Autodesk Inventor part; units mm, degrees
ref_plane "YZ Plane" through (0, 0, 0) normal (1, 0, 0) x (0, 1, 0)
ref_plane "XZ Plane" through (0, 0, 0) normal (0, 1, 0) x (-1, 0, 0)
ref_plane "XY Plane" through (0, 0, 0) normal (0, 0, 1) x (1, 0, 0)
sketch "スケッチ1" plane through (0, 0, 0) normal (0, 0, 1) x (1, 0, 0)
  line L0 (-20, -5) -> (20, -5)
  line L1 (20, -5) -> (20, 5)
  line L2 (20, 5) -> (-20, 5)
  line L3 (-20, 5) -> (-20, -5)
  line L4 (-20, -5) -> (20, 5) construction
  line L5 (20, -5) -> (-20, 5) construction
  point P0 (0, 0)
  dimension "d0" = 40
  dimension "d1" = 10
extrude "押し出し1" add sketch "スケッチ1" along normal mid plane 3
sketch "スケッチ2" plane through (-20, -5, 1.5) normal (-1, 0, 0) x (0, 0, 1)
  line L0 (0, 0) -> (0, 10)
  line L1 (-3, 3) -> (0, 3)
  line L2 (0, 3) -> (0, 7)
  line L3 (0, 7) -> (-3, 7)
  line L4 (-3, 7) -> (-3, 3)
  line L5 (-3, 3) -> (0, 7) construction
  line L6 (0, 3) -> (-3, 7) construction
  point P0 (-1.5, 5)
  dimension "d4" = 4
extrude "押し出し2" add sketch "スケッチ2" along normal blind 5
sketch "スケッチ3" plane through (20, -5, 1.5) normal (1, 0, 0) x (0, 0, -1)
  line L0 (3, 7) -> (0, 7)
  line L1 (0, 3) -> (3, 3)
  line L2 (3, 10) -> (0, 10)
  line L3 (0, 0) -> (0, 10)
  line L4 (0, 0) -> (3, 0)
  line L5 (3, 10) -> (3, 0)
  point P0 (1.5, 5)
extrude "押し出し3" add sketch "スケッチ3" along normal blind 5 contours L5 L1 L3 L0
fillet "フィレット1" radius 1 8 edges at (25, 2, 0) (25, 0, 1.5) (25, 0, -1.5) (25, -2, 0) (-25, 0, 1.5) (-25, 0, -1.5) (-25, 2, 0) (-25, -2, 0)
chamfer "面取り1" distance 2 angle 45 1 edges at (0, -5, 1.5)
properties part number "刃"
Can you work these out from the model? Positions are in its coordinate system, mm. A direction names the side the tool comes from. Round coordinates to 2 decimals unless told otherwise and drop trailing zeros. Order: outer loops, then holes, each group sorted by start corner. A loop starts at its lowest first (then second) coordinate and runs counter-clockwise, first axis right, second up. Notation, with made-up numbers: M 69.5,40 L 127.5,40 A27 cw 127.5,78 Z; hole C -12,49 d4. An arc over 180 degrees is marked long. Use a Markdown table: item, result.
1) I'm going to push flat-ended pins straight in: P1, Ø0.9, axis at y = -3, z = -0.5, coming from the +X side; P2, Ø0.9, axis at x = 21.5, z = 0.5, coming from the +Y side; P3, Ø0.9, axis at y = -3, z = -0.5, coming from the -X side. Where does each tip first touch, or does it pass through?
Geometry says:
| item | result |
|---|---|
| P1 | stops at x = 20 |
| P2 | stops at y = 2 |
| P3 | stops at x = -20 |
2) Imagine slicing it at C-C (x = 21). List the corners of the cut face in (y, z) for me, then the cut area to 3 significant figures.
Geometry says:
| item | result |
|---|---|
| outline | M -2,-1.5 L 2,-1.5 L 2,1.5 L -2,1.5 Z |
| area | 12.0 mm² |
3) Imagine slicing it at A-A (x = 7.5). List the corners of the cut face in (y, z) for me.
Geometry says:
| item | result |
|---|---|
| outline | M -5,-1.5 L 5,-1.5 L 5,1.5 L -3,1.5 L -5,-0.5 Z |
4) If I drill on line 1 along X through (y, z) = (-2.5, 1.35); line 2 along Y through (x, z) = (-22, 0.1); line 3 along Y through (x, z) = (-2.5, 0.85), over which ranges is the centre line in solid material (lowest first)?
Geometry says:
| item | result |
|---|---|
| line 1 | x = -20 to 20 |
| line 2 | y = -2 to 2 |
| line 3 | y = -3.65 to 5 |
5) On a 3-axis mill with a long thin cutter (end or side, diameter ignored), from which of +Z, -Z, +X, -X, +Y, -Y can I reach the whole of each face in a straight line? I mean faces 1 (the face through (-22, -2, 0)), 2 (the face through (20, -3, 0)), 3 (the face through (-22, 2, 0)). Say none if no direction works.
Geometry says:
| item | result |
|---|---|
| face 1 | +Z, -Z, -X, -Y |
| face 2 | +Z, -Z, +X, -Y |
| face 3 | +Z, -Z, -X, +Y |
6) Imagine slicing it at B-B (y = 4.25). List the corners of the cut face in (x, z) for me.
Geometry says:
| item | result |
|---|---|
| outline | M -20,-1.5 L 20,-1.5 L 20,1.5 L -20,1.5 Z |
